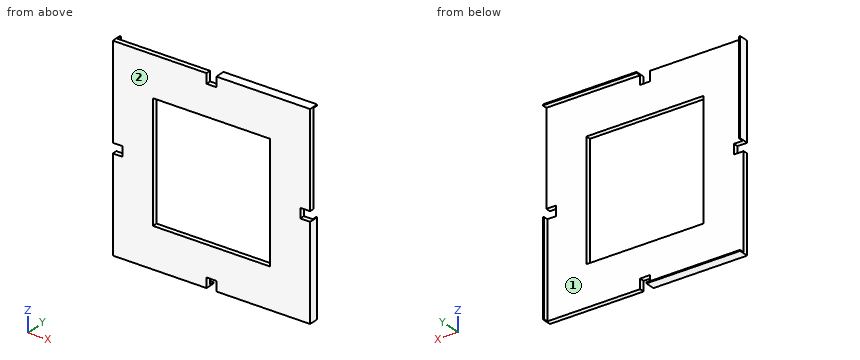
```python
from build123d import *

# Parameters (mm, degrees)
SKETCH1_W           = 120
SKETCH1_H           = 120
BOSS_EXTRUDE1_DEPTH = 5
SKETCH2_W           = 96
SKETCH2_H           = 1
SKETCH2_W_2         = 1
SKETCH2_H_2         = 96
BOSS_EXTRUDE2_DEPTH = 5


with BuildPart() as part:
    # Sketch1 → Boss-Extrude1 (new body)
    with BuildSketch(Plane(origin=(0, 0, 0), x_dir=(1, 0, 0), z_dir=(0, 1, 0))):
        Polygon((101, -101), (5, -101), (5, -91), (-5, -91), (-5, -101), (-101, -101), (-101, -5), (-91, -5), (-91, 5), (-101, 5), (-101, 101), (-5, 101), (-5, 91), (5, 91), (5, 101), (101, 101), (101, 5), (91, 5), (91, -5), (101, -5), align=None)
        Rectangle(SKETCH1_W, SKETCH1_H, mode=Mode.SUBTRACT)
    extrude(amount=BOSS_EXTRUDE1_DEPTH)

    # Sketch2 → Boss-Extrude2 (add)
    with BuildSketch(Plane(origin=(0, 5, 0), x_dir=(1, 0, 0), z_dir=(0, 1, 0))):
        with Locations((53, -100.5)):
            Rectangle(SKETCH2_W, SKETCH2_H)
        with Locations((-100.5, -53)):
            Rectangle(SKETCH2_W_2, SKETCH2_H_2)
        with Locations((-53, 100.5)):
            Rectangle(SKETCH2_W, SKETCH2_H)
        with Locations((100.5, 53)):
            Rectangle(SKETCH2_W_2, SKETCH2_H_2)
    extrude(amount=BOSS_EXTRUDE2_DEPTH)


solid = part.part
```
Read the model definition and answer for the solid it produces. Units are mm, in the model's axes. Face numbers are marked on the shaded views. A direction names the side the tool comes from. Coordinates: 2 decimals unless noted, no trailing zeros. Write each loop counter-clockwise with the first axis right and the second up, starting at its lowest first coordinate (ties: lowest second). Pieces come first, ordered by that corner, then holes. Notation, with made-up numbers: (41.25, -32) - (48.25, -32) arc R29 ccw to (48.25, -4) - close; hole circle Ø3 at (-11, 28.5). An arc over 180 degrees is marked (long way). Answer as a JSON object with one key per item and string values. Group by question number.
1. Each of these flat-tipped pins is pushed along its axis until it touches: P1, Ø1.5, axis at y = 7, z = -43.5, coming from the -X side; P2, Ø5, axis at x = -28, z = -72.5, coming from the +Y side; P3, Ø5.5, axis at y = 8, z = 40, coming from the +X side. Where does it stop, or does it pass through?
2. Which of the six approach directions +Z, -Z, +X, -X, +Y, -Y give full straight-line access (tool end or side, diameter ignored) to the marked faces 1 and 2?
3. A cutting plane is placed at A-A (x = 28). Determine the outline of the cut face in (y, z), plus the area to 3 significant figures.
4. Consider L1, parallel to X at y = 2.25, z = 4; L2, parallel to Z at x = -9.5, y = 0.5. Determine where each line is inside the solid, lowest interval first. Write a range as [from, to].
5. A cutting plane is placed at B-B (z = -38). Determine the outline of the cut face in (x, y).
6. A cutting plane is placed at C-C (y = 2.5). Determine the outline of the cut face in (x, z), plus the area to 3 significant figures.
7. A cutting plane is placed at D-D (x = 71.5). Determine the outline of the cut face in (y, z), plus the area to 4 significant figures.
Worked out:
{
 "1": {"P1": "stops at x = 100", "P2": "stops at y = 5", "P3": "stops at x = -100"},
 "2": {"face 1": "+Y", "face 2": "+Z, -Z, +X, -X, -Y"},
 "3": {"outline": "(0, -101) - (5, -101) - (5, -60) - (0, -60) - close; (0, 60) - (5, 60) - (5, 100) - (10, 100) - (10, 101) - (0, 101) - close", "area": "415 mm²"},
 "4": {"L1": "x = [-91, -60], [60, 91]", "L2": "z = [-101, -60], [60, 101]"},
 "5": {"outline": "(-101, 0) - (-60, 0) - (-60, 5) - (-101, 5) - close; (60, 0) - (101, 0) - (101, 10) - (100, 10) - (100, 5) - (60, 5) - close"},
 "6": {"outline": "(-101, -101) - (-5, -101) - (-5, -91) - (5, -91) - (5, -101) - (101, -101) - (101, -5) - (91, -5) - (91, 5) - (101, 5) - (101, 101) - (5, 101) - (5, 91) - (-5, 91) - (-5, 101) - (-101, 101) - (-101, 5) - (-91, 5) - (-91, -5) - (-101, -5) - close; hole (-60, -60) - (60, -60) - (60, 60) - (-60, 60) - close", "area": "26,000 mm²"},
 "7": {"outline": "(0, -101) - (5, -101) - (5, 100) - (10, 100) - (10, 101) - (0, 101) - close", "area": "1,015 mm²"}
}
